```python
from build123d import *

# Parameters (mm, degrees)
ESQUISSE6_W              = 98
ESQUISSE6_H              = 130
BOSS_EXTRU_4_DEPTH       = 48
COQUE7_T                 = 1.6
EXTRU_MINCE1_DEPTH       = 45
EXTRU_MINCE1_DEPTH_BACK  = 1.6
ESQUISSE7_W              = 104.8
ESQUISSE7_H              = 136.8
ESQUISSE7_W_2            = 98
ESQUISSE7_H_2            = 130
ESQUISSE13_W             = 85
ESQUISSE13_H             = 63.5
ENL_V_MAT_EXTRU_10_DEPTH = 8
ESQUISSE16_R             = 1.5
BOSS_EXTRU_9_DEPTH       = 9
ESQUISSE17_R             = 3
BOSS_EXTRU_10_DEPTH      = 2.54
ESQUISSE17_4_R           = 3
ENL_V_MAT_EXTRU_11_DEPTH = 6
CONG_5_R                 = 3
CONG_6_R                 = 1
ESQUISSE22_W             = 45
ESQUISSE22_H             = 11
ENL_V_MAT_EXTRU_12_DEPTH = 6
CONG_7_R                 = 1
BOSS_EXTRU_15_DEPTH      = 20
BOSS_EXTRU_16_DEPTH      = 20
ENL_V_MAT_EXTRU_14_DEPTH = 19
ENL_V_MAT_EXTRU_15_DEPTH = 19
CONG_8_R                 = 1
ESQUISSE17_7_R           = 1.9
BOSS_EXTRU_18_DEPTH      = 6


with BuildPart() as part:
    # Esquisse6 → Boss.-Extru.4 (new body)
    with BuildSketch(Plane(origin=(0, 0, 0), x_dir=(1, 0, 0), z_dir=(0, 1, 0))):
        Rectangle(ESQUISSE6_W, ESQUISSE6_H)
    extrude(amount=BOSS_EXTRU_4_DEPTH)

    # Coque7
    coque7_openings = [part.faces().sort_by_distance(p)[0] for p in [
        (0, 48, 0),
    ]]
    offset(amount=COQUE7_T, openings=coque7_openings, kind=Kind.INTERSECTION)

    # Esquisse13 → Enl_v. mat.-Extru.10 (cut)
    with BuildSketch(Plane(origin=(0, -1.6, 0), x_dir=(-1, 0, 0), z_dir=(0, -1, 0))):
        with Locations((0, -22.25)):
            Rectangle(ESQUISSE13_W, ESQUISSE13_H)
    extrude(amount=-ENL_V_MAT_EXTRU_10_DEPTH, mode=Mode.SUBTRACT)


with BuildPart() as body_2:
    # Esquisse7 → Extru.-Mince1 (new, two sides: drawn at the far end of the back side and taken through both)
    with BuildSketch(Plane(origin=(0, 0, 0), x_dir=(1, 0, 0), z_dir=(0, 1, 0)).offset(-EXTRU_MINCE1_DEPTH_BACK)):
        Rectangle(ESQUISSE7_W, ESQUISSE7_H)
        Rectangle(ESQUISSE7_W_2, ESQUISSE7_H_2, mode=Mode.SUBTRACT)
    extrude(amount=EXTRU_MINCE1_DEPTH + EXTRU_MINCE1_DEPTH_BACK)


    add(part.part)  # Boss.-Extru.9 merges part
    # Esquisse16 → Boss.-Extru.9 (add)
    with BuildSketch(Plane(origin=(0, 0, 0), x_dir=(1, 0, 0), z_dir=(0, 1, 0))):
        with Locations(Location((43.125, 23.25, 0), (0, 0, 270))):
            Circle(ESQUISSE16_R)
        with Locations(Location((43.125, -61, 0), (0, 0, 270))):
            Circle(ESQUISSE16_R)
        with Locations(Location((-43.125, -61, 0), (0, 0, 270))):
            Circle(ESQUISSE16_R)
        with Locations(Location((-43.125, 23.25, 0), (0, 0, 270))):
            Circle(ESQUISSE16_R)
    extrude(amount=BOSS_EXTRU_9_DEPTH)

    # Esquisse17 → Boss.-Extru.10 (add)
    with BuildSketch(Plane(origin=(0, 0, 0), x_dir=(1, 0, 0), z_dir=(0, 1, 0))):
        with Locations(Location((16.5, 32, 0), (0, 0, 270))):
            Circle(ESQUISSE17_R)
        with Locations(Location((16.5, 50, 0), (0, 0, 270))):
            Circle(ESQUISSE17_R)
        with Locations(Location((-8.5, 50, 0), (0, 0, 270))):
            Circle(ESQUISSE17_R)
        with Locations(Location((-8.5, 32, 0), (0, 0, 270))):
            Circle(ESQUISSE17_R)
    extrude(amount=BOSS_EXTRU_10_DEPTH)

    # Esquisse17_4 → Enl_v. mat.-Extru.11 (cut)
    with BuildSketch(Plane(origin=(0, 0, 0), x_dir=(1, 0, 0), z_dir=(0, 1, 0))):
        with Locations(Location((0, 41, 0), (0, 0, 270))):
            Circle(ESQUISSE17_4_R)
    extrude(amount=-ENL_V_MAT_EXTRU_11_DEPTH, mode=Mode.SUBTRACT)

    # Cong_5
    cong_5_edges = [body_2.edges().sort_by_distance(p)[0] for p in [
        (-52.4, -1.6, 0),
        (0, -1.6, 68.4),
        (52.4, -1.6, 0),
        (52.4, 21.7, 68.4),
        (-52.4, 21.7, 68.4),
        (-52.4, 21.7, -68.4),
        (52.4, 21.7, -68.4),
        (0, -1.6, -68.4),
    ]]
    fillet(cong_5_edges, radius=CONG_5_R)

    # Cong_6
    cong_6_edges = [body_2.edges().sort_by_distance(p)[0] for p in [
        (42.5, -0.8, 54),
        (42.5, -0.8, -9.5),
        (-42.5, -0.8, -9.5),
        (-42.5, -0.8, 54),
    ]]
    fillet(cong_6_edges, radius=CONG_6_R)

    # Esquisse22 → Enl_v. mat.-Extru.12 (cut)
    with BuildSketch(Plane.XY.offset(68.4)):
        with Locations((0, 27.5)):
            Rectangle(ESQUISSE22_W, ESQUISSE22_H)
    extrude(amount=-ENL_V_MAT_EXTRU_12_DEPTH, mode=Mode.SUBTRACT)

    # Cong_7
    cong_7_edges = [body_2.edges().sort_by_distance(p)[0] for p in [
        (0, 22, 65),
        (22.5, 27.5, 65),
        (0, 33, 65),
        (-22.5, 27.5, 65),
        (-22.5, 22, 66.7),
        (-22.5, 33, 66.7),
        (0, 33, 68.4),
        (22.5, 33, 66.7),
        (22.5, 27.5, 68.4),
        (22.5, 22, 66.7),
        (-22.5, 27.5, 68.4),
        (0, 22, 68.4),
    ]]
    fillet(cong_7_edges, radius=CONG_7_R)

    # Esquisse3D2 → Boss.-Extru.15 (add, symmetric)
    with BuildSketch(Plane(origin=(49, 46, 0), x_dir=(-0.7071067811865488, 0.7071067811865464, 0), z_dir=(0, 0, -1))):
        Polygon((0, 0), (-1.414213562, -1.414213562), (1.414213562, -1.414213562), (2.828427125, 0), (1.414213562, 1.414213562), align=None)
    boss_extru_15 = extrude(amount=BOSS_EXTRU_15_DEPTH, both=True)

    # Sym_trie1: Boss.-Extru.15 across plane
    add(boss_extru_15.mirror(Plane(origin=(0, 0, 0), x_dir=(0, 0, 1), z_dir=(1, 0, 0))))

    # Esquisse3D4 → Boss.-Extru.16 (add, symmetric)
    with BuildSketch(Plane(origin=(0, 48, -65), x_dir=(0, -1, 0), z_dir=(-1, 0, 0))):
        Polygon((0, 0), (0, 2), (2, 2), (4, 0), (2, 0), align=None)
    boss_extru_16 = extrude(amount=BOSS_EXTRU_16_DEPTH, both=True)

    # Esquisse3D6 → Enl_v. mat.-Extru.14 (cut, symmetric)
    with BuildSketch(Plane(origin=(50.6, 48, 0), x_dir=(0, -1, 0), z_dir=(0, 0, -1))):
        Polygon((0, 0), (3, 0), (1.5, 1.322875656), align=None)
    enl_v_mat_extru_14 = extrude(amount=ENL_V_MAT_EXTRU_14_DEPTH, both=True, mode=Mode.SUBTRACT)

    # Sym_trie2: Enl_v. mat.-Extru.14 across plane
    add(enl_v_mat_extru_14.mirror(Plane(origin=(0, 0, 0), x_dir=(0, 0, 1), z_dir=(1, 0, 0))), mode=Mode.SUBTRACT)

    # Sym_trie3: Boss.-Extru.16 across plane
    add(boss_extru_16.mirror(Plane.XY))

    # Esquisse3D7 → Enl_v. mat.-Extru.15 (cut, symmetric)
    with BuildSketch(Plane(origin=(0, 48, -66.6), x_dir=(0, -1, 0), z_dir=(-1, 0, 0))):
        Polygon((0, 0), (3, 0), (1.5, 1.322875656), align=None)
    enl_v_mat_extru_15 = extrude(amount=ENL_V_MAT_EXTRU_15_DEPTH, both=True, mode=Mode.SUBTRACT)

    # Sym_trie5: Enl_v. mat.-Extru.15 across plane
    add(enl_v_mat_extru_15.mirror(Plane.XY), mode=Mode.SUBTRACT)

    # Cong_8
    cong_8_edges = [body_2.edges().sort_by_distance(p)[0] for p in [
        (0, -1.6, -44),
    ]]
    fillet(cong_8_edges, radius=CONG_8_R)

    # Esquisse17_7 → Boss.-Extru.18 (add)
    with BuildSketch(Plane(origin=(0, 0, 0), x_dir=(1, 0, 0), z_dir=(0, 1, 0))):
        with Locations(Location((16.5, 32, 0), (0, 0, 270))):
            Circle(ESQUISSE17_7_R)
        with Locations(Location((16.5, 50, 0), (0, 0, 270))):
            Circle(ESQUISSE17_7_R)
        with Locations(Location((-8.5, 32, 0), (0, 0, 270))):
            Circle(ESQUISSE17_7_R)
        with Locations(Location((-8.5, 50, 0), (0, 0, 270))):
            Circle(ESQUISSE17_7_R)
    extrude(amount=BOSS_EXTRU_18_DEPTH)


solid = body_2.part
```
Model file for the job. Use its own axes, mm. A direction names the side the tool comes from. Coordinates: 2 decimals unless noted, no trailing zeros. Write each loop counter-clockwise with the first axis right and the second up, starting at its lowest first coordinate (ties: lowest second). Pieces come first, ordered by that corner, then holes. Notation, with made-up numbers: (88, -6) - (140, -6) arc R26 ccw to (140, 29) - close; hole circle Ø10 at (33, -38.5). An arc over 180 degrees is marked (long way). One line per item, written item: value. Start each with the question number.
1. Slice it at D-D (x = 9.5). Count the separate pieces of the cut face and the enclosed holes in it, plus the area to 3 significant figures.
2. Slice it at B-B (x = -37). Write the cut outline in (y, z), plus the area to 3 significant figures.
3. Probe line 1 (X direction, y = 13.5, z = -50); line 2 (Z direction, x = 16, y = 16); line 3 (Y direction, x = 34, z = -16). List the from-to ranges inside material, lowest first. Write a range as from..to.
4. Mould opens along Y. For faces 5 (the flat face through (49, 24, 1)), 6 (the cylindrical face through (-8.4, 1.3, -35)), 7 (the cylindrical face through (0.69, -0.74, -67.5)) say: released by +Y, released by -Y, zero draft, split by the parting line, or undercut.
5. Slice it at A-A (z = -1). Write the cut outline in (x, y), plus the area to 3 significant figures.
6. Tool access for faces 1 (the flat face through (-1, 24, -65)), 2 (the flat face through (-50.6, 46, 43)), 3 (the flat face through (50.6, 46, 43)), 4 (the cylindrical face through (-44.59, 4.44, -23.58)): list every direction of +Z, -Z, +X, -X, +Y, -Y with a clear straight run to the whole face (end or side of a thin tool).
7. Slice it at C-C (y = 42.5). Write the cut outline in (x, z).
8. Flat gauge pins, fed straight in: pin 1 (1.5 mm diameter, centred on x = 37.5, y = 46, fed in from -Z); pin 2 (0.6 mm diameter, centred on y = 47, z = -0.5, fed in from +X); pin 3 (1.8 mm diameter, centred on y = -1, z = 18, fed in from -X); pin 4 (10 mm diameter, centred on x = -22, y = 31.5, fed in from +Z). Where does each tip first touch, or does it go through?
Answers below:
1. separate pieces: 3
1. enclosed holes: 0
1. area: 399 mm^2
2. outline: (-1.6, -65.4) arc R3 ccw to (1.4, -68.4) - (45, -68.4) - (45, -66.6) - (48, -66.6) - (48, -65) - (0, -65) - (0, -9.5) - (-1.6, -9.5) - close; (-1.6, 54) - (0, 54) - (0, 65) - (48, 65) - (48, 66.6) - (45, 66.6) - (45, 68.4) - (1.4, 68.4) arc R3 ccw to (-1.6, 65.4) - close
2. area: 429 mm^2
3. line 1: x = -52.4..-49, 49..52.4
3. line 2: z = -68.4..-65, 65..68.4
3. line 3: y = -1.6..0
4. face 5: undercut
4. face 6: zero draft
4. face 7: released by -Y
5. outline: (-52.4, 1.4) arc R3 ccw to (-49.4, -1.6) - (-42.5, -1.6) - (-42.5, 0) - (-49, 0) - (-49, 44) - (-47, 46) - (-47, 48) - (-50.6, 48) - (-49.28, 46.5) - (-50.6, 45) - (-52.4, 45) - close; (42.5, -1.6) - (49.4, -1.6) arc R3 ccw to (52.4, 1.4) - (52.4, 45) - (50.6, 45) - (49.28, 46.5) - (50.6, 48) - (47, 48) - (47, 46) - (49, 44) - (49, 0) - (42.5, 0) - close
5. area: 351 mm^2
6. face 1: none
6. face 2: +Z, -Z, -X, +Y
6. face 3: +Z, -Z, +X, +Y
6. face 4: +Y
7. outline: (-52.4, -65.4) arc R3 ccw to (-49.4, -68.4) - (49.4, -68.4) arc R3 ccw to (52.4, -65.4) - (52.4, 65.4) arc R3 ccw to (49.4, 68.4) - (-49.4, 68.4) arc R3 ccw to (-52.4, 65.4) - close; hole (-49, -65) - (49, -65) - (49, 65) - (-49, 65) - close
8. pin 1: stops at z = -66.6
8. pin 2: stops at x = 49.98
8. pin 3: stops at x = -52
8. pin 4: stops at z = 68.4
